Could you check a few things on this model? Use its own coordinates, in mm. Face numbers are marked on the shaded views. A direction names the side the tool comes from. Coordinates: 2 decimals unless noted, no trailing zeros. Order: outer loops, then holes, each group sorted by start corner. A loop starts at its lowest first (then second) coordinate and runs counter-clockwise, first axis right, second up.
```python
from build123d import *

# Parameters (mm, degrees)
BOSS_EXTRUDE1_DEPTH = 4
SKETCH1_R           = 1.375
CUT_EXTRUDE1_DEPTH  = 4


with BuildPart() as part:
    # Sketch2 → Boss-Extrude1 (new body)
    with BuildSketch(Plane(origin=(0, 0, 0), x_dir=(1, 0, 0), z_dir=(0, 1, 0))):
        Polygon((17.875, 15.25), (21.875, 15.25), (21.875, -15.25), (17.875, -15.25), (17.875, -17.88), (-17.875, -17.88), (-17.875, -15.25), (-21.875, -15.25), (-21.875, 15.25), (-17.875, 15.25), (-17.875, 17.88), (17.875, 17.88), align=None)
    extrude(amount=BOSS_EXTRUDE1_DEPTH)

    # Sketch1 → Cut-Extrude1 (cut)
    with BuildSketch(Plane(origin=(0, 0, 0), x_dir=(1, 0, 0), z_dir=(0, 1, 0))):
        with Locations(Location((-15.25, 15.25, 0), (0, 0, 270))):
            Circle(SKETCH1_R)
        with Locations(Location((15.25, 15.25, 0), (0, 0, 270))):
            Circle(SKETCH1_R)
        with Locations(Location((15.25, -15.25, 0), (0, 0, 270))):
            Circle(SKETCH1_R)
        with Locations(Location((-15.25, -15.25, 0), (0, 0, 270))):
            Circle(SKETCH1_R)
    extrude(amount=CUT_EXTRUDE1_DEPTH, mode=Mode.SUBTRACT)


solid = part.part
```
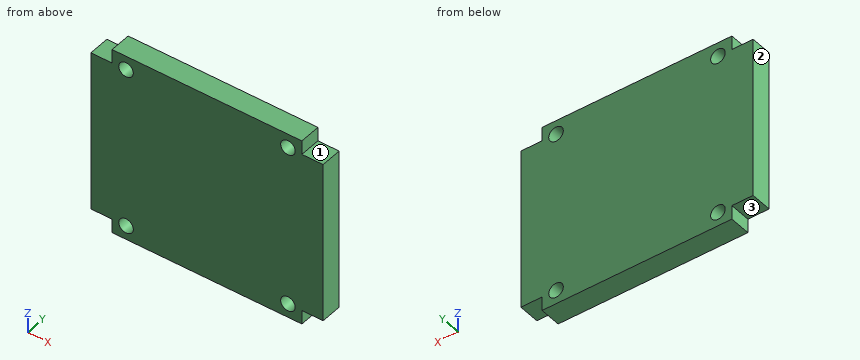
Item 1: Which directions (+Z, -Z, +X, -X, +Y, -Y) give clear straight access to the entire face, cutting with the end or side of a thin tool? Please do the marked faces 1, 2 and 3.
Item 2: I need wall thicknesses on line 1 (Z direction, x = 14.5, y = 2.3); line 2 (X direction, y = 3.25, z = 15) (3 decimals); line 3 (X direction, y = 2.25, z = -16) (3 decimals). Which ranges of each line are inside material? Lowest first, please.
Item 3: Suppose I cut it at B-B (y = 0.9). List the corners of the cut face in (x, z) for me (3 decimals).
Item 4: Suppose I cut it at A-A (x = -15.25). List the corners of the cut face in (y, z) for me (3 decimals), and give its area (3 significant figures).
Item 5: For pin 1 Ø1.5 at (x, z) = (8, -2.5) entering from -Y; pin 2 Ø1.2 at (x, y) = (19, 2) entering from +Z; pin 3 Ø1.3 at (y, z) = (1.5, -17) entering from -X (3 decimals); pin 4 Ø2 at (y, z) = (1, 17) entering from +X (3 decimals), each with a flat end and sliding along its axis, tell me the tip position at first contact or that it passes through.
Geometry results:
1. face 1: +Z, +X, +Y, -Y
1. face 2: +Z, -Z, -X, +Y, -Y
1. face 3: -Z, -X, +Y, -Y
2. line 1: z = -17.88 to -16.4, -14.1 to 14.1, 16.4 to 17.88
2. line 2: x = -21.875 to -16.602, -13.898 to 13.898, 16.602 to 21.875
2. line 3: x = -17.875 to -16.402, -14.098 to 14.098, 16.402 to 17.875
3. outline: (-21.875, -15.25) - (-17.875, -15.25) - (-17.875, -17.88) - (17.875, -17.88) - (17.875, -15.25) - (21.875, -15.25) - (21.875, 15.25) - (17.875, 15.25) - (17.875, 17.88) - (-17.875, 17.88) - (-17.875, 15.25) - (-21.875, 15.25) - close; hole circle Ø2.75 at (-15.25, -15.25); hole circle Ø2.75 at (-15.25, 15.25); hole circle Ø2.75 at (15.25, -15.25); hole circle Ø2.75 at (15.25, 15.25)
4. outline: (0, -17.88) - (4, -17.88) - (4, -16.625) - (0, -16.625) - close; (0, -13.875) - (4, -13.875) - (4, 13.875) - (0, 13.875) - close; (0, 16.625) - (4, 16.625) - (4, 17.88) - (0, 17.88) - close
4. area: 121 mm2
5. pin 1: stops at y = 0
5. pin 2: stops at z = 15.25
5. pin 3: stops at x = -17.875
5. pin 4: stops at x = 17.875
